```python
from build123d import *

# Parameters (mm, degrees)
SKETCH1_W           = 6
SKETCH1_H           = 6
BOSS_EXTRUDE1_DEPTH = 1.5
SKETCH2_W           = 6
SKETCH2_H           = 3
BOSS_EXTRUDE2_DEPTH = 1.5
SKETCH3_W           = 6
SKETCH3_H           = 6
BOSS_EXTRUDE4_DEPTH = 1.5
SKETCH4_W           = 6
SKETCH4_H           = 3
BOSS_EXTRUDE5_DEPTH = 1.5
SKETCH5_W           = 6
SKETCH5_H           = 6
BOSS_EXTRUDE6_DEPTH = 1.5


with BuildPart() as part:
    # Sketch1 → Boss-Extrude1 (new body)
    with BuildSketch(Plane.XY):
        with Locations((0, -1.5)):
            Rectangle(SKETCH1_W, SKETCH1_H)
    extrude(amount=BOSS_EXTRUDE1_DEPTH)

    # Sketch2 → Boss-Extrude2 (add)
    with BuildSketch(Plane(origin=(0, 0, 0), x_dir=(-1, 0, 0), z_dir=(0, 0, -1))):
        Rectangle(SKETCH2_W, SKETCH2_H)
    extrude(amount=BOSS_EXTRUDE2_DEPTH)

    # Sketch3 → Boss-Extrude4 (add)
    with BuildSketch(Plane(origin=(0, 0, -1.5), x_dir=(-1, 0, 0), z_dir=(0, 0, -1))):
        with Locations((0, -1.5)):
            Rectangle(SKETCH3_W, SKETCH3_H)
    extrude(amount=BOSS_EXTRUDE4_DEPTH)

    # Sketch4 → Boss-Extrude5 (add)
    with BuildSketch(Plane(origin=(0, 0, -3), x_dir=(-1, 0, 0), z_dir=(0, 0, -1))):
        with Locations((0, -3)):
            Rectangle(SKETCH4_W, SKETCH4_H)
    extrude(amount=BOSS_EXTRUDE5_DEPTH)

    # Sketch5 → Boss-Extrude6 (add)
    with BuildSketch(Plane(origin=(0, 0, -4.5), x_dir=(-1, 0, 0), z_dir=(0, 0, -1))):
        with Locations((0, -1.5)):
            Rectangle(SKETCH5_W, SKETCH5_H)
    extrude(amount=BOSS_EXTRUDE6_DEPTH)


solid = part.part
```
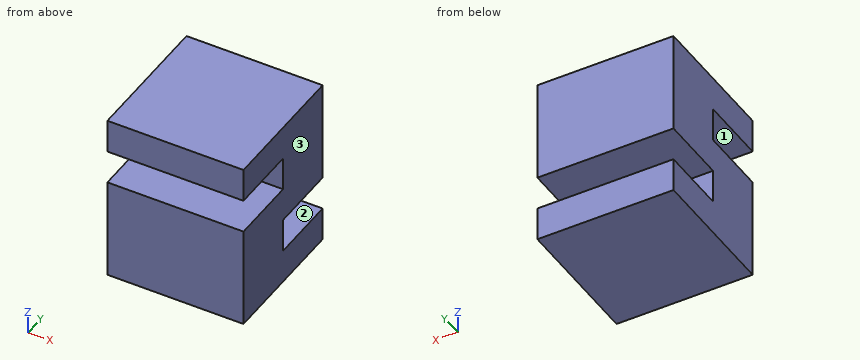
Verification items for the finished model (mm, model axes). Face numbers are marked on the shaded views. A direction names the side the tool comes from. Coordinates: 2 decimals unless noted, no trailing zeros. Order: outer loops, then holes, each group sorted by start corner. A loop starts at its lowest first (then second) coordinate and runs counter-clockwise, first axis right, second up. Notation, with made-up numbers: (75.5, 57.25) - (80.5, 57.25) arc R22 cw to (80.5, 71.25) - close; hole circle Ø10 at (33.5, 33.25). An arc over 180 degrees is marked (long way). Return JSON: item names as keys, results as strings.
(1) Go/stop test with a flat-tipped pin: pin 1 (0.8 mm diameter, centred on x = -1, z = -1, fed in from -Y). Record where the tip stops, or that it passes through.
Filled sheet:
{"pin 1": "stops at y = -1.5"}
(2) Section check A-A, the plane y = -2.15. Record the cut outline in (x, z), and give its area (3 significant figures).
Filled sheet:
{"outline": "(-3, -6) - (3, -6) - (3, -1.5) - (-3, -1.5) - close; (-3, 0) - (3, 0) - (3, 1.5) - (-3, 1.5) - close", "area": "36.0 mm^2"}
(3) Section check C-C, the plane z = -4. Record the cut outline in (x, y).
Filled sheet:
{"outline": "(-3, -4.5) - (3, -4.5) - (3, -1.5) - (-3, -1.5) - close"}
(4) Section check B-B, the plane x = 1.35. Record the cut outline in (y, z).
Filled sheet:
{"outline": "(-4.5, -6) - (1.5, -6) - (1.5, -4.5) - (-1.5, -4.5) - (-1.5, -3) - (1.5, -3) - (1.5, 1.5) - (-4.5, 1.5) - (-4.5, 0) - (-1.5, 0) - (-1.5, -1.5) - (-4.5, -1.5) - close"}
(5) Thickness scan on line 1 along Z through (x, y) = (-0.9, -3.25); line 2 along Z through (x, y) = (1.7, 0.05); line 3 along Y through (x, z) = (-2.65, -3.5). Record the ranges inside material, lowest first.
Filled sheet:
{"line 1": "z = -6 to -1.5, 0 to 1.5", "line 2": "z = -6 to -4.5, -3 to 1.5", "line 3": "y = -4.5 to -1.5"}
(6) Access from +Z, -Z, +X, -X, +Y, -Y to the whole of each face (thin tool, end or side, straight path). Record for the marked faces 1, 2 and 3.
Filled sheet:
{"face 1": "+X, -X, -Y", "face 2": "+X, -X, +Y", "face 3": "+Z, -Z, +X, +Y, -Y"}
